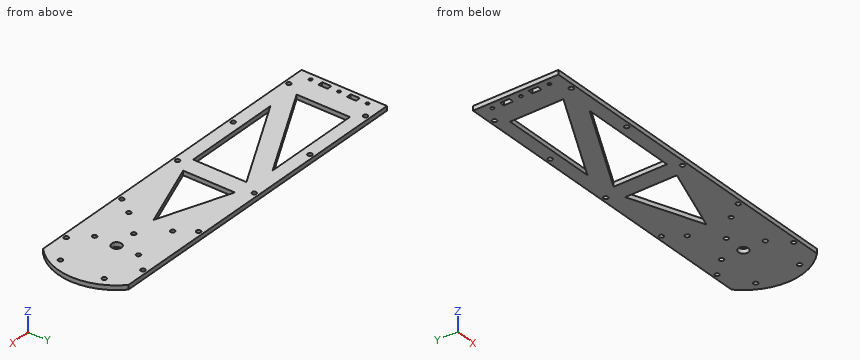
from build123d import *

# Parameters (mm, degrees)
SKETCH_1_R      = 1.5
SKETCH_1_R_2    = 4.5
SKETCH_1_R_3    = 2
SKETCH_1_W      = 4.4
SKETCH_1_H      = 8.4
EXTRUDE_1_DEPTH = 4


with BuildPart() as part:
    # 草图1 → 凸台-拉伸1 (new body)
    with BuildSketch(Plane.XY):
        with BuildLine():
            Line((-6, 39), (-6, -39))
            Line((-6, -39), (296.024297356, -39))
            ThreePointArc((296.024297356, -39), (313.091901454, 0), (296.024297356, 39))
            Line((296.024297356, 39), (-6, 39))
        make_face()
        Circle(SKETCH_1_R, mode=Mode.SUBTRACT)
        with Locations(Location((0, 26, 0), (0, 0, 180))):
            Circle(SKETCH_1_R, mode=Mode.SUBTRACT)
        with Locations((0, -26)):
            Circle(SKETCH_1_R, mode=Mode.SUBTRACT)
        with Locations((260, 0)):
            Circle(SKETCH_1_R_2, mode=Mode.SUBTRACT)
        with Locations((260, 20)):
            Circle(SKETCH_1_R_3, mode=Mode.SUBTRACT)
        with Locations((240, 0)):
            Circle(SKETCH_1_R_3, mode=Mode.SUBTRACT)
        with Locations((300, 20)):
            Circle(SKETCH_1_R_3, mode=Mode.SUBTRACT)
        with Locations((300, -20)):
            Circle(SKETCH_1_R_3, mode=Mode.SUBTRACT)
        with Locations((220, 20)):
            Circle(SKETCH_1_R_3, mode=Mode.SUBTRACT)
        with Locations((220, -20)):
            Circle(SKETCH_1_R_3, mode=Mode.SUBTRACT)
        with Locations((260, -20)):
            Circle(SKETCH_1_R_3, mode=Mode.SUBTRACT)
        with Locations((274, -35)):
            Circle(SKETCH_1_R_3, mode=Mode.SUBTRACT)
        with Locations((209, -35)):
            Circle(SKETCH_1_R_3, mode=Mode.SUBTRACT)
        with Locations((144, -35)):
            Circle(SKETCH_1_R_3, mode=Mode.SUBTRACT)
        with Locations((79, -35)):
            Circle(SKETCH_1_R_3, mode=Mode.SUBTRACT)
        with Locations((14, -35)):
            Circle(SKETCH_1_R_3, mode=Mode.SUBTRACT)
        with Locations((209, 35)):
            Circle(SKETCH_1_R_3, mode=Mode.SUBTRACT)
        with Locations((144, 35)):
            Circle(SKETCH_1_R_3, mode=Mode.SUBTRACT)
        with Locations((79, 35)):
            Circle(SKETCH_1_R_3, mode=Mode.SUBTRACT)
        with Locations((14, 35)):
            Circle(SKETCH_1_R_3, mode=Mode.SUBTRACT)
        with Locations((274, 35)):
            Circle(SKETCH_1_R_3, mode=Mode.SUBTRACT)
        with Locations((0, 13)):
            Rectangle(SKETCH_1_W, SKETCH_1_H, mode=Mode.SUBTRACT)
        with Locations((0, -13)):
            Rectangle(SKETCH_1_W, SKETCH_1_H, mode=Mode.SUBTRACT)
        Polygon((22, -21.606262732), (112.268773645, 27), (22, 27), align=None, mode=Mode.SUBTRACT)
        Polygon((45.731226355, -27), (136, -27), (136, 21.606262732), align=None, mode=Mode.SUBTRACT)
        Polygon((152, -23.568232368), (216.644294496, 0), (152, 23.568232368), align=None, mode=Mode.SUBTRACT)
    extrude(amount=EXTRUDE_1_DEPTH)


solid = part.part
Work out the finished part from the listing and answer in its coordinate system (mm). Give positions to 0.01 mm unless a question says otherwise; leave off trailing zeros. Loops run counter-clockwise (first coordinate to the right, second up) from the corner with the lowest first, then second, coordinate; pieces in that order, holes last. Notation, with made-up numbers: (20.5, 59.5) - (67.5, 59.5) arc R24 cw to (67.5, 82.5) - close; hole circle Ø2 at (86, -13.75). An arc over 180 degrees is marked (long way). Answer in a Markdown table with one row per item. Add a question column.
Q1. The part is cut by section A-A (x = 119.5). Determine the outline of the cut face in (y, z).
Q2. Consider line 1 along Y through (x, z) = (14, 2.25); line 2 along Y through (x, z) = (0, 2.6); line 3 along Y through (x, z) = (260.5, 0.8). Determine where each line is inside the solid, lowest interval first.
Q3. The part is cut by section C-C (z = 0.8). State how many separate pieces and enclosed holes the cut face has, and give its area (3 significant figures).
Q4. The part is cut by section D-D (x = 196.5). Determine the outline of the cut face in (y, z), and give its area (3 significant figures).
Q5. The part is cut by section B-B (x = 52.5). Determine the outline of the cut face in (y, z).
Solution:
| question | item | result |
|---|---|---|
| 1 | outline | (-39, 0) - (-27, 0) - (-27, 4) - (-39, 4) - close; (12.72, 0) - (39, 0) - (39, 4) - (12.72, 4) - close |
| 2 | line 1 | y = -39 to -37, -33 to 33, 37 to 39 |
| 2 | line 2 | y = -39 to -27.5, -24.5 to -17.2, -8.8 to -1.5, 1.5 to 8.8, 17.2 to 24.5, 27.5 to 39 |
| 2 | line 3 | y = -39 to -21.94, -18.06 to -4.47, 4.47 to 18.06, 21.94 to 39 |
| 3 | separate pieces | 1 |
| 3 | enclosed holes | 26 |
| 3 | area | 18,200 mm² |
| 4 | outline | (-39, 0) - (-7.34, 0) - (-7.34, 4) - (-39, 4) - close; (7.34, 0) - (39, 0) - (39, 4) - (7.34, 4) - close |
| 4 | area | 253 mm² |
| 5 | outline | (-39, 0) - (-27, 0) - (-27, 4) - (-39, 4) - close; (-23.36, 0) - (-5.18, 0) - (-5.18, 4) - (-23.36, 4) - close; (27, 0) - (39, 0) - (39, 4) - (27, 4) - close |
